```python
from build123d import *

# Parameters (mm, degrees)
F0_W     = 381
F0_H     = 279.4
F7_DEPTH = 12.7


with BuildPart() as f3:
    # F0 (on Top) → F3 section 0
    with BuildSketch(Plane.XY):
        Polygon((203.2, 152.4), (-203.2, 152.4), (-190.5, 139.7), (190.5, 139.7), align=None)
    # F2 (on offset) → F3 section 1
    with BuildSketch(Plane.XY.offset(254)):
        Polygon((266.7, 190.5), (-266.7, 190.5), (-254, 177.8), (254, 177.8), align=None)
    loft()

    # F0 (on Top) → F4 section 0
    with BuildSketch(Plane.XY):
        Polygon((-190.5, 139.7), (-203.2, 152.4), (-203.2, -152.4), (-190.5, -139.7), align=None)
    # F2 (on offset) → F4 section 1
    with BuildSketch(Plane.XY.offset(254)):
        Polygon((-254, 177.8), (-266.7, 190.5), (-266.7, -190.5), (-254, -177.8), align=None)
    loft()

    # F2 (on offset) → F5 section 0
    with BuildSketch(Plane.XY.offset(254)):
        Polygon((-254, -177.8), (-266.7, -190.5), (266.7, -190.5), (254, -177.8), align=None)
    # F0 (on Top) → F5 section 1
    with BuildSketch(Plane.XY):
        Polygon((-190.5, -139.7), (-203.2, -152.4), (203.2, -152.4), (190.5, -139.7), align=None)
    loft()

    # F2 (on offset) → F6 section 0
    with BuildSketch(Plane.XY.offset(254)):
        Polygon((266.7, -190.5), (266.7, 190.5), (254, 177.8), (254, -177.8), align=None)
    # F0 (on Top) → F6 section 1
    with BuildSketch(Plane.XY):
        Polygon((203.2, -152.4), (203.2, 152.4), (190.5, 139.7), (190.5, -139.7), align=None)
    loft()

    # F0 (on Top) → F7 (join)
    with BuildSketch(Plane.XY):
        Polygon((203.2, 152.4), (-203.2, 152.4), (-190.5, 139.7), (190.5, 139.7), align=None)
        Polygon((-190.5, 139.7), (-203.2, 152.4), (-203.2, -152.4), (-190.5, -139.7), align=None)
        Polygon((-190.5, -139.7), (-203.2, -152.4), (203.2, -152.4), (190.5, -139.7), align=None)
        Polygon((203.2, -152.4), (203.2, 152.4), (190.5, 139.7), (190.5, -139.7), align=None)
        Rectangle(F0_W, F0_H)
    extrude(amount=F7_DEPTH)


solid = f3.part
```
Geometry: final body of the model. Coordinates: model frame, mm. Coordinates: 2 decimals unless noted, no trailing zeros. Answer in a Markdown table with one row per item. Add a question column.
Q1. Line query: L1, parallel to Z at x = -67, y = 85; L2, parallel to X at y = -21, z = 240; L3, parallel to X at y = 125, z = 199.5 (3 decimals). Output: solid intervals per line, ascending.
Q2. Mould query, pull axis X, two halves, no side actions, for faces 1 (the flat face through (-3, -2, 0)), 2 (the flat face through (-3, 2, 12.7)). Classes: released by +X, released by -X, zero draft, split by the parting line, or undercut.
Q3. Contact query for flat-ended pins moving along their axis: P1, Ø3, axis at x = -2.5, y = -138.5, coming from the +Z side; P2, Ø1, axis at y = 112, z = 34.5, coming from the -X side; P3, Ø3, axis at y = 42.5, z = 60, coming from the -X side (3 decimals). Output: stop coordinate, or through.
Completed:
| question | item | result |
|---|---|---|
| 1 | L1 | z = 0 to 12.7 |
| 1 | L2 | x = -263.2 to -250.5, 250.5 to 263.2 |
| 1 | L3 | x = -253.075 to -240.375, 240.375 to 253.075 |
| 2 | face 1 | zero draft |
| 2 | face 2 | undercut |
| 3 | P1 | stops at z = 12.7 |
| 3 | P2 | stops at x = -211.95 |
| 3 | P3 | stops at x = -218.575 |
